Design review of the part built by this model. Coordinates are the model's own, in mm. A direction names the side the tool comes from. Coordinates: 2 decimals unless noted, no trailing zeros. Write each loop counter-clockwise with the first axis right and the second up, starting at its lowest first coordinate (ties: lowest second). Pieces come first, ordered by that corner, then holes. Notation, with made-up numbers: (55.5, 79.5) -> (68.5, 79.5) arc R20 cw to (68.5, 116.5) -> close; hole circle Ø2 at (70, -28.5). An arc over 180 degrees is marked (long way). One line per question, with ' | ' between items. Start each with the question number.
Q1. Wall thickness on probe 1 along Y at (x, z) = (45, 0.6); probe 2 along Z at (x, y) = (14, 2.75); probe 3 along Y at (x, z) = (20, -6.75): over which ranges is each line inside the solid? List them lowest first.
Q2. Add section B-B on z = -7. State the section outline as (x, y) points.
Q3. Draft analysis for pull direction Y (two halves, no side actions). For faces 1 (the cylindrical face through (53.498, 0.187, 0.493)), 2 (the cylindrical face through (22.58, -0.08, -8.8)), 3 (the cylindrical face through (-1.717, 0.541, 0.493)), 4 (the flat face through (22.8, -8.5, 0.5)), state which applies: pulls with the +Y half, pulls with the -Y half, needs draft (parallel to the pull), parting line crosses it, or undercut.
Q4. Add section A-A on x = 19. State the section outline as (y, z) points.
Q5. For faces 5 (the flat face through (25.25, 0.9, -0.5)), 6 (the flat face through (23, -7, -8)), 7 (the flat face through (17.778, 2.581, -6.916)), list the 3-axis set-ups (+Z, -Z, +X, -X, +Y, -Y) from which the entire face can be reached by the end or side of a thin tool; tool diameter is ignored.
Q6. For P1, Ø4, axis at y = 0, z = -7, coming from the -X side; P2, Ø3, axis at x = 1, y = -4.5, coming from the -Z side; P3, Ø4, axis at y = 6, z = -2.5, coming from the -X side; P4, Ø3, axis at x = 0, y = 0, coming from the +Z side, all flat-tipped, find the tip position at first contact; note any pin that passes through.
Q7. Add section C-C on y = 0. State the section outline as (x, z) points.
Q8. Add section D-D on y = -4. State the section outline as (x, z) points, and give its area (4 significant figures).
from build123d import *

# Parameters (mm, degrees)
BOSS_EXTRUDE1_DEPTH      = 1
M3_CLEARANCE_HOLE1_D     = 3.6
M3_CLEARANCE_HOLE1_DEPTH = 1
BOSS_EXTRUDE2_DEPTH      = 15.5
M3_CLEARANCE_HOLE2_D     = 3.6


with BuildPart() as part:
    # Sketch1 → Boss-Extrude1 (new body)
    with BuildSketch(Plane.XY):
        with BuildLine():
            Line((0, 8.5), (45, 8.5))
            ThreePointArc((45, 8.5), (53.5, 0), (45, -8.5))
            Line((45, -8.5), (0, -8.5))
            ThreePointArc((0, -8.5), (-8.5, 0), (0, 8.5))
        make_face()
    extrude(amount=BOSS_EXTRUDE1_DEPTH)

    # M3 Clearance Hole1
    with Locations(Plane.XY.offset(1)):
        with Locations((0, 0), (45, 0)):
            Hole(M3_CLEARANCE_HOLE1_D / 2, depth=M3_CLEARANCE_HOLE1_DEPTH)

    # Sketch4 → Boss-Extrude2 (add)
    with BuildSketch(Plane(origin=(0, 8.5, 0), x_dir=(1, 0, 0), z_dir=(0, 1, 0))):
        Polygon((19.75, 0), (19.75, 1), (15.75, 13), (29.25, 13), (25.25, 1), (25.25, 0), align=None)
    extrude(amount=-BOSS_EXTRUDE2_DEPTH)

    # M3 Clearance Hole2 (through all)
    with Locations(Plane(origin=(0, 0, 0), x_dir=(0, 0, -1), z_dir=(-1, 0, 0))):
        with Locations((7, 0)):
            Hole(M3_CLEARANCE_HOLE2_D / 2)


solid = part.part
Output values:
1) probe 1: y = -8.5 to -1.8, 1.8 to 8.5 | probe 2: z = 0 to 1 | probe 3: y = -7 to -1.78, 1.78 to 8.5
2) outline: (17.75, -7) -> (27.25, -7) -> (27.25, -1.8) -> (17.75, -1.8) -> close; (17.75, 1.8) -> (27.25, 1.8) -> (27.25, 8.5) -> (17.75, 8.5) -> close
3) face 1: parting line crosses it | face 2: undercut | face 3: undercut | face 4: pulls with the -Y half
4) outline: (-8.5, 0) -> (8.5, 0) -> (8.5, 1) -> (-8.5, 1) -> close; (-7, -13) -> (8.5, -13) -> (8.5, -3.25) -> (-7, -3.25) -> close; hole circle Ø3.6 at (0, -7)
5) face 5: +X, +Y, -Y | face 6: -Z, +X, -X, -Y | face 7: -X, +Y, -Y
6) P1: stops at x = 17.08 | P2: stops at z = 0 | P3: stops at x = 18.58 | P4: passes through
7) outline: (-8.5, 0) -> (-1.8, 0) -> (-1.8, 1) -> (-8.5, 1) -> close; (1.8, 0) -> (19.75, 0) -> (19.75, -1) -> (18.35, -5.2) -> (26.65, -5.2) -> (25.25, -1) -> (25.25, 0) -> (43.2, 0) -> (43.2, 1) -> (1.8, 1) -> close; (15.75, -13) -> (29.25, -13) -> (27.85, -8.8) -> (17.15, -8.8) -> close; (46.8, 0) -> (53.5, 0) -> (53.5, 1) -> (46.8, 1) -> close
8) outline: (-7.5, 0) -> (19.75, 0) -> (19.75, -1) -> (15.75, -13) -> (29.25, -13) -> (25.25, -1) -> (25.25, 0) -> (52.5, 0) -> (52.5, 1) -> (-7.5, 1) -> close | area: 179.5 mm2
